Input: part model. Units: mm. Frame: model coordinates. Face numbers are marked on the shaded views. A direction names the side the tool comes from. Round coordinates to 2 decimals unless told otherwise and drop trailing zeros. Loops run counter-clockwise (first coordinate to the right, second up) from the corner with the lowest first, then second, coordinate; pieces in that order, holes last. Notation, with made-up numbers: (73, 78.5) - (121, 78.5) arc R13 ccw to (121, 94.5) - close; hole circle Ø10 at (50.25, 25). An arc over 180 degrees is marked (long way). One line per question, with ' | ' between items. Start each with the question number.
Item 1: Section B-B, the plane y = 39. Return loops of the section in (x, z).
Item 2: Section A-A, the plane x = 32.5. Return loops of the section in (y, z), plus the area to 3 significant figures.
Item 3: Section C-C, the plane z = 12. Return loops of the section in (x, y), plus the area to 3 significant figures.
Item 4: Material intervals for line 1 along Y through (x, z) = (0, 4); line 2 along Y through (x, z) = (26, 6); line 3 along X through (y, z) = (48, 12.75), sorted ascending.
Item 5: First-contact query: pin 1 (2 mm diameter, centred on y = 32, z = 7.5, fed in from +X); pin 2 (2 mm diameter, centred on x = 19, z = 3.5, fed in from -Y); pin 3 (1 mm diameter, centred on y = 17.5, z = 5.5, fed in from -X); pin 4 (4.5 mm diameter, centred on y = 46, z = 10, fed in from +X). Flat tips, straight axial feed; report the tip coordinate or a pass-through.
Item 6: Draft query along X for the marked faces 1, 2 and 3. Return one class per face: pulls with the +X half, pulls with the -X half, needs draft (parallel to the pull), parting line crosses it, or undercut.
Item 7: Set-up query: the marked faces 4, 5 and 6. Return all of +Z, -Z, +X, -X, +Y, -Y with unobstructed straight access to the full face (end or side cutting, diameter ignored); none if empty.
Item 8: Section D-D, the plane y = 32. Return loops of the section in (x, z), plus the area to 3 significant figures.
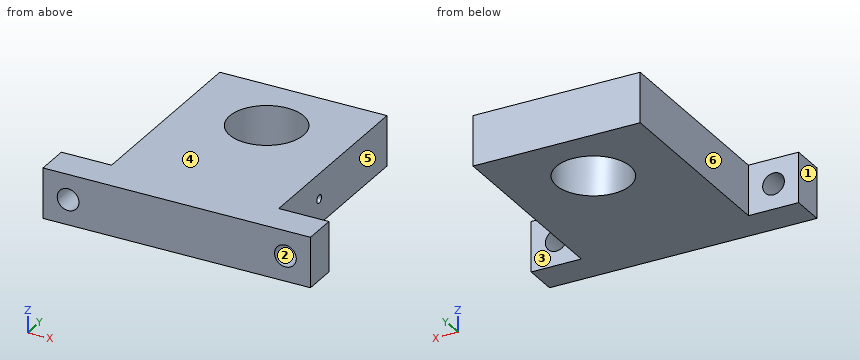
```python
from build123d import *

# Parameters (mm, degrees)
SKETCH1_R           = 11.0998
BOSS_EXTRUDE1_DEPTH = 15
SKETCH2_R           = 3.25
CUT_EXTRUDE1_DEPTH  = 73.765855395
SKETCH3_R           = 1.25
CUT_EXTRUDE2_DEPTH  = 4.5


with BuildPart() as part:
    # Sketch1 → Boss-Extrude1 (new body)
    with BuildSketch(Plane.XY):
        Polygon((-40, 0), (40, 0), (40, 10), (25, 10), (25, 68.9056), (-25, 68.9056), (-25, 10), (-40, 10), align=None)
        with Locations((0, 48.9056)):
            Circle(SKETCH1_R, mode=Mode.SUBTRACT)
    extrude(amount=BOSS_EXTRUDE1_DEPTH)

    # Sketch2 → Cut-Extrude1 (cut, through all)
    with BuildSketch(Plane(origin=(0, 10, 0), x_dir=(1, 0, 0), z_dir=(0, 1, 0))):
        with Locations(Location((-32.5, -7.5, 0), (0, 0, 180))):
            Circle(SKETCH2_R)
        with Locations(Location((32.5, -7.5, 0), (0, 0, 180))):
            Circle(SKETCH2_R)
    extrude(amount=-CUT_EXTRUDE1_DEPTH, mode=Mode.SUBTRACT)

    # Sketch3 → Cut-Extrude2 (cut)
    with BuildSketch(Plane(origin=(25, 0, 0), x_dir=(0, 0, -1), z_dir=(1, 0, 0))):
        with Locations(Location((-7.5, 32, 0), (0, 0, 90))):
            Circle(SKETCH3_R)
    extrude(amount=-CUT_EXTRUDE2_DEPTH, mode=Mode.SUBTRACT)


solid = part.part
```
Return value:
1) outline: (-25, 0) - (-5.01, 0) - (-5.01, 15) - (-25, 15) - close; (5.01, 0) - (25, 0) - (25, 15) - (5.01, 15) - close
2) outline: (0, 0) - (10, 0) - (10, 4.25) - (0, 4.25) - close; (0, 10.75) - (10, 10.75) - (10, 15) - (0, 15) - close | area: 85.0 mm2
3) outline: (-40, 0) - (40, 0) - (40, 10) - (25, 10) - (25, 68.91) - (-25, 68.91) - (-25, 10) - (-40, 10) - close; hole circle Ø22.2 at (0, 48.91) | area: 3,360 mm2
4) line 1: 0 to 37.81, 60.01 to 68.91 | line 2: 0 to 10 | line 3: -25 to -11.06, 11.06 to 25
5) pin 1: x = 20.5 | pin 2: y = 0 | pin 3: x = -25 | pin 4: x = 25
6) face 1: pulls with the -X half | face 2: undercut | face 3: needs draft
7) face 4: +Z, +X, -X, +Y, -Y | face 5: +Z, -Z, +X, +Y | face 6: +Z, -Z, -X, +Y
8) outline: (-25, 0) - (25, 0) - (25, 6.25) - (20.5, 6.25) - (20.5, 8.75) - (25, 8.75) - (25, 15) - (-25, 15) - close | area: 739 mm2
